Job drawing, mm, ordinate dimensions from the low corner. One solid piece. A direction names the side the tool comes from. Give positions to 0.01 mm unless a question says otherwise; leave off trailing zeros. Write each loop counter-clockwise with the first axis right and the second up, starting at its lowest first coordinate (ties: lowest second). Pieces come first, ordered by that corner, then holes. Notation, with made-up numbers: (41.5, 4) - (68.5, 4) arc R21 ccw to (68.5, 42) - close; hole circle Ø1 at (-15, 55.5). An arc over 180 degrees is marked (long way). Put each result on its own line as item: value. Start each with the question number.
1. Tool access for the marked faces 4 and 5: list every direction of +Z, -Z, +X, -X, +Y, -Y with a clear straight run to the whole face (end or side of a thin tool).
2. Cut at D-D on z = 8.5. Give the number of separate pieces and of enclosed holes in the cut face.
3. Wall check: line 1 (Z direction, x = 16.5, y = 1.5) (1 decimal); line 2 (Z direction, x = 29, y = 0.75) (1 decimal); line 3 (X direction, y = 4.25, z = 23) (1 decimal). Give the ranges that are in metal, low to high.
4. Cut at A-A on z = 19.5. List the corners of the cut face in (x, y).
5. Cut at C-C on y = 0.5. List the corners of the cut face in (x, z) (1 decimal).
6. Cut at B-B on x = 23. List the corners of the cut face in (y, z).
7. Drop flat-ended pins along their axis: pin 1 (1.5 mm diameter, centred on x = 18, y = 2.5, fed in from +Z); pin 2 (1.5 mm diameter, centred on x = 20.5, y = 4, fed in from -Z); pin 3 (1.5 mm diameter, centred on x = 29.5, y = 2.5, fed in from -Z). Give the stop position or say it passes through.
8. Mould opens along Z. For the marked faces 1, 2 and 3 say: +Z half, -Z half, draft (parallel to the pull), parting line (faces both ways), or undercut.
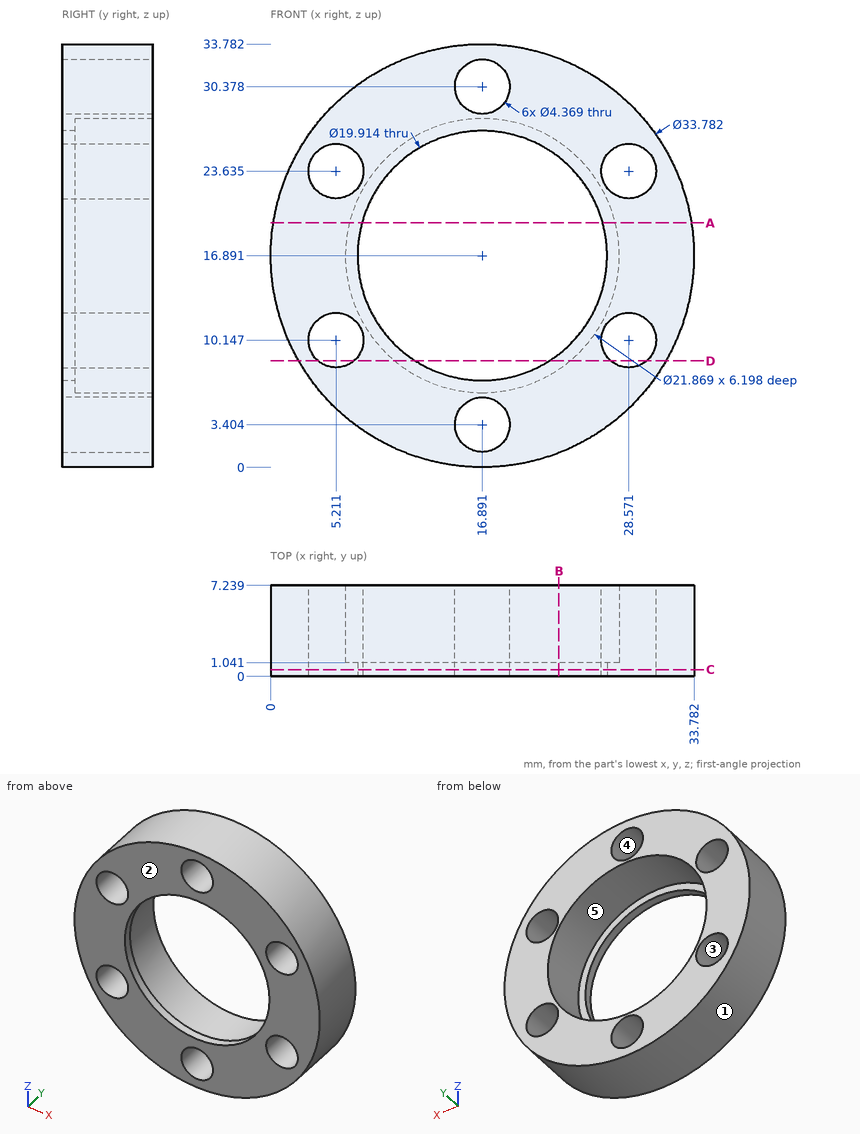
Report:
1. face 4: +Y, -Y
1. face 5: +Y
2. separate pieces: 4
2. enclosed holes: 0
3. line 1: z = 0 to 1.3, 5.6 to 6, 27.8 to 28.2, 32.5 to 33.8
3. line 2: z = 5.1 to 8, 12.3 to 21.5, 25.8 to 28.7
3. line 3: x = 1.1 to 3.1, 7.3 to 7.8, 26 to 26.5, 30.7 to 32.6
4. outline: (0.2, 0) - (7.28, 0) - (7.28, 1.04) - (6.27, 1.04) - (6.27, 7.24) - (0.2, 7.24) - close; (26.5, 0) - (33.58, 0) - (33.58, 7.24) - (27.51, 7.24) - (27.51, 1.04) - (26.5, 1.04) - close
5. outline: circle Ø33.8 at (16.9, 16.9); hole circle Ø4.4 at (5.2, 10.1); hole circle Ø4.4 at (5.2, 23.6); hole circle Ø19.9 at (16.9, 16.9); hole circle Ø4.4 at (16.9, 3.4); hole circle Ø4.4 at (16.9, 30.4); hole circle Ø4.4 at (28.6, 10.1); hole circle Ø4.4 at (28.6, 23.6)
6. outline: (0, 1.14) - (7.24, 1.14) - (7.24, 7.82) - (1.04, 7.82) - (1.04, 9.03) - (0, 9.03) - close; (0, 24.75) - (1.04, 24.75) - (1.04, 25.96) - (7.24, 25.96) - (7.24, 32.64) - (0, 32.64) - close
7. pin 1: stops at z = 33.78
7. pin 2: stops at z = 0.24
7. pin 3: stops at z = 4.86
8. face 1: parting line
8. face 2: draft
8. face 3: undercut
